Geometry check sheet. Reference: the model listing, model coordinates, mm. A direction names the side the tool comes from. Coordinates: 2 decimals unless noted, no trailing zeros. Answer in a Markdown table with one row per item. Add a question column.
1. Set-up check for faces 1 (the flat face through (25, 15, 1)), 2 (the cylindrical face through (-77.26, 13.17, 24.33)): record each of +Z, -Z, +X, -X, +Y, -Y from which the full face is reachable in a straight line by a thin tool's end or side.
2. Scan lines: L1, parallel to Z at x = 0, y = 13.65; L2, parallel to Z at x = 0, y = 0.75; L3, parallel to Z at x = 0, y = 7.6. Record each from-to range of solid material in increasing order. Write a range as from..to.
3. Depth check by flat-ended pin: P1, Ø8, axis at x = -39.5, z = 52, coming from the -Y side; P2, Ø12, axis at y = 2, z = 59, coming from the +X side; P3, Ø4, axis at x = -1, z = 2, coming from the -Y side. Enter the tip coordinate at first touch or a pass-through.
4. Mould release check, pull along X, two halves, no side actions. Record for faces 3 (the flat face through (18, -7.5, 12)), 4 (the cylindrical face through (-12.465, 13.479, -56.133)), 5 (the conical face through (16.734, 3.694, 75.359)): pulls with the +X half, pulls with the -X half, needs draft (parallel to the pull), parting line crosses it, or undercut.
```python
from build123d import *

# Parameters (mm, degrees)
SKETCH2_R           = 71
BOSS_EXTRUDE1_DEPTH = 11
SKETCH12_R          = 57.5
SKETCH12_R_2        = 23.75
CUT_EXTRUDE8_DEPTH  = 1
CUT_EXTRUDE9_START  = -10
SKETCH10_R          = 85
SKETCH10_R_2        = 81
CUT_EXTRUDE9_DEPTH  = 10
SKETCH14_R          = 57.5
SKETCH14_R_2        = 23.75
BOSS_EXTRUDE2_DEPTH = 1
SKETCH15_R          = 81
BOSS_EXTRUDE3_DEPTH = 4
SKETCH16_R          = 57.5
SKETCH16_R_2        = 23.75
CUT_EXTRUDE11_DEPTH = 2
SKETCH17_W          = 29
SKETCH17_H          = 10.11
SKETCH17_H_2        = 35.11
BOSS_EXTRUDE4_DEPTH = 3


with BuildPart() as part:
    # Sketch1 → Revolve1 (revolve)
    with BuildSketch(Plane.XY, mode=Mode.PRIVATE) as revolve1_sk:
        Polygon((0, 12), (0, 15), (85, 15), (85, 10.5), (84, 10.5), (77, 3.5), (77, 0), (71, 0), (71, 12), (23.75, 12), (23.75, -7.5), (21.25, -7.5), (21.25, 6), (6.5, 6), (6.5, 9), (0, 9), align=None)
    revolve(revolve1_sk.sketch.rotate(Axis((0, 12, 0), (0, -1, 0)), 180), axis=Axis((0, 12, 0), (0, -1, 0)))

    # Sketch2 → Boss-Extrude1 (add)
    with BuildSketch(Plane.XZ.offset(-12)):
        with Locations(Location((0, 0, 0), (0, 0, 180))):
            Circle(SKETCH2_R)
        Polygon((0, 70.292395274), (-60.875, 35.146197637), (-60.875, -35.146197637), (0, -70.292395274), (60.875, -35.146197637), (60.875, 35.146197637), align=None, mode=Mode.SUBTRACT)
    extrude(amount=BOSS_EXTRUDE1_DEPTH)

    # Sketch12 → Cut-Extrude8 (cut)
    with BuildSketch(Plane.XZ.offset(-12)):
        Circle(SKETCH12_R)
        with Locations(Location((0, 0, 0), (0, 0, 180))):
            Circle(SKETCH12_R_2, mode=Mode.SUBTRACT)
    extrude(amount=-CUT_EXTRUDE8_DEPTH, mode=Mode.SUBTRACT)

    # Sketch10 → Cut-Extrude9 (cut)
    with BuildSketch(Plane(origin=(0, 15, 0), x_dir=(1, 0, 0), z_dir=(0, 1, 0)).offset(CUT_EXTRUDE9_START)):
        Circle(SKETCH10_R)
        with Locations(Location((0, 0, 0), (0, 0, 180))):
            Circle(SKETCH10_R_2, mode=Mode.SUBTRACT)
    extrude(amount=CUT_EXTRUDE9_DEPTH, mode=Mode.SUBTRACT)

    # Sketch14 → Boss-Extrude2 (add)
    with BuildSketch(Plane(origin=(0, 13, 0), x_dir=(-1, 0, 0), z_dir=(0, -1, 0))):
        with Locations(Location((0, 0, 0), (0, 0, 180))):
            Circle(SKETCH14_R)
        Circle(SKETCH14_R_2, mode=Mode.SUBTRACT)
    extrude(amount=-BOSS_EXTRUDE2_DEPTH)

    # Sketch15 → Boss-Extrude3 (add)
    with BuildSketch(Plane(origin=(0, 15, 0), x_dir=(1, 0, 0), z_dir=(0, 1, 0))):
        with Locations(Location((0, 0, 0), (0, 0, 180))):
            Circle(SKETCH15_R)
    extrude(amount=BOSS_EXTRUDE3_DEPTH)

    # Sketch16 → Cut-Extrude11 (cut)
    with BuildSketch(Plane.XZ.offset(-13)):
        Circle(SKETCH16_R)
        with Locations(Location((0, 0, 0), (0, 0, 180))):
            Circle(SKETCH16_R_2, mode=Mode.SUBTRACT)
    extrude(amount=-CUT_EXTRUDE11_DEPTH, mode=Mode.SUBTRACT)

    # Sketch17 → Boss-Extrude4 (add)
    with BuildSketch(Plane(origin=(0, 19, 0), x_dir=(1, 0, 0), z_dir=(0, 1, 0))):
        with Locations((-48.833648901, -5.055)):
            Rectangle(SKETCH17_W, SKETCH17_H)
        with Locations((-48.833648901, 17.555)):
            Rectangle(SKETCH17_W, SKETCH17_H_2)
        with Locations((48.416351099, -5.055)):
            Rectangle(SKETCH17_W, SKETCH17_H)
        with Locations((48.416351099, 17.555)):
            Rectangle(SKETCH17_W, SKETCH17_H_2)
    extrude(amount=BOSS_EXTRUDE4_DEPTH)


solid = part.part
```
Results found:
| question | item | result |
|---|---|---|
| 1 | face 1 | -Y |
| 1 | face 2 | +Y, -Y |
| 2 | L1 | z = -81..-57.5, -23.75..23.75, 57.5..81 |
| 2 | L2 | z = -77..-71, -23.75..-21.25, 21.25..23.75, 71..77 |
| 2 | L3 | z = -81..-70.29, -23.75..-6.5, 6.5..23.75, 70.29..81 |
| 3 | P1 | stops at y = 1 |
| 3 | P2 | stops at x = 58.14 |
| 3 | P3 | stops at y = 9 |
| 4 | face 3 | needs draft |
| 4 | face 4 | undercut |
| 4 | face 5 | parting line crosses it |
